Here's how the part is built. I have some questions about the finished solid (model axes, mm). A direction names the side the tool comes from. Round coordinates to 2 decimals unless told otherwise and drop trailing zeros. Write each loop counter-clockwise with the first axis right and the second up, starting at its lowest first coordinate (ties: lowest second). Pieces come first, ordered by that corner, then holes. Notation, with made-up numbers: (-26, -39.75) -> (26, -39.75) arc R34 cw to (26, -6.75) -> close; hole circle Ø9 at (11, 65). An arc over 180 degrees is marked (long way). Answer in a Markdown table with one row per item.
from build123d import *

# Parameters (mm, degrees)
F1_DEPTH = 7.5
F2_R     = 1.5
F3_DEPTH = 0.4910000058
F4_R     = 1.5
F5_DEPTH = 0.4910000058


with BuildPart() as f1:
    # F0 (on Right) → F1 (new body, symmetric)
    with BuildSketch(Plane.YZ):
        with BuildLine():
            Line((0, 0), (0, 30))
            ThreePointArc((0, 30), (-0.2450000029, 30.2450000029), (-0.4900000058, 30))
            Line((-0.4900000058, 30), (-0.4900000058, -0.4900000058))
            Line((-0.4900000058, -0.4900000058), (30, -0.4900000058))
            ThreePointArc((30, -0.4900000058), (30.2450000029, -0.2450000029), (30, 0))
            Line((30, 0), (0, 0))
        make_face()
    extrude(amount=F1_DEPTH, both=True)

    # F2 (on face) → F3 (cut, through all)
    with BuildSketch(Plane(origin=(0, 0, 0), x_dir=(-1, 0, 0), z_dir=(0, 1, 0))):
        with Locations((0, 20)):
            Circle(F2_R)
        with Locations((0, 10)):
            Circle(F2_R)
    extrude(amount=-F3_DEPTH, mode=Mode.SUBTRACT)

    # F4 (on face) → F5 (cut, through all)
    with BuildSketch(Plane.XY):
        with Locations((0, 20)):
            Circle(F4_R)
        with Locations((0, 10)):
            Circle(F4_R)
    extrude(amount=-F5_DEPTH, mode=Mode.SUBTRACT)


solid = f1.part
1) I want a section at D-D, the plane x = 3.25. List the corners of the cut face in (y, z) for me (3 decimals).
Response:
| item | result |
|---|---|
| outline | (-0.49, -0.49) -> (30, -0.49) arc R0.245 ccw to (30, 0) -> (0, 0) -> (0, 30) arc R0.245 ccw to (-0.49, 30) -> close |
2) I want a section at C-C, the plane x = 0. List the corners of the cut face in (y, z) for me (3 decimals), and give its area (3 significant figures).
Response:
| item | result |
|---|---|
| outline | (-0.49, -0.49) -> (8.5, -0.49) -> (8.5, 0) -> (0, 0) -> (0, 8.5) -> (-0.49, 8.5) -> close; (-0.49, 11.5) -> (0, 11.5) -> (0, 18.5) -> (-0.49, 18.5) -> close; (-0.49, 21.5) -> (0, 21.5) -> (0, 30) arc R0.245 ccw to (-0.49, 30) -> close; (11.5, -0.49) -> (18.5, -0.49) -> (18.5, 0) -> (11.5, 0) -> close; (21.5, -0.49) -> (30, -0.49) arc R0.245 ccw to (30, 0) -> (21.5, 0) -> close |
| area | 23.9 mm^2 |
3) We'd pull the mould along Y, two halves only. Please class faces 3 (the face through (-0.195, 21.487, -0.242)), 4 (the face through (0, -0.49, 15)), 5 (the face through (-0.325, 8.536, -0.242)), 6 (the face through (0, 15, -0.49)): +Y half, -Y half, draft (parallel to the pull), parting line (faces both ways), or undercut.
Response:
| item | result |
|---|---|
| face 3 | undercut |
| face 4 | -Y half |
| face 5 | undercut |
| face 6 | draft |
4) I want a section at A-A, the plane y = 20. List the corners of the cut face in (x, z) for me.
Response:
| item | result |
|---|---|
| outline | (-7.5, -0.49) -> (-1.5, -0.49) -> (-1.5, 0) -> (-7.5, 0) -> close; (1.5, -0.49) -> (7.5, -0.49) -> (7.5, 0) -> (1.5, 0) -> close |
5) I need wall thicknesses on line 1 (Y direction, x = 0, z = -0.25); line 2 (Z direction, x = 0.5, y = 27.5). Which ranges of each line are inside material? Lowest first, please. Write a range as [from, to].
Response:
| item | result |
|---|---|
| line 1 | y = [-0.49, 8.5], [11.5, 18.5], [21.5, 30.24] |
| line 2 | z = [-0.49, 0] |
6) Which directions (+Z, -Z, +X, -X, +Y, -Y) give clear straight access to the entire face, cutting with the end or side of a thin tool? Please do faces 1 (the face through (0, 15, 0)), 2 (the face through (0.195, -0.242, 21.487)).
Response:
| item | result |
|---|---|
| face 1 | +Z, +X, -X, +Y |
| face 2 | +Y, -Y |
7) For pin 1 (4 mm diameter, centred on x = 0, z = 20, fed in from +Y); pin 2 (1 mm diameter, centred on x = 5, y = 22.5, fed in from +Z); pin 3 (2.5 mm diameter, centred on x = 0, y = 20, fed in from +Z), each with a flat end and sliding along its axis, tell me the tip position at first contact or that it passes through.
Response:
| item | result |
|---|---|
| pin 1 | stops at y = 0 |
| pin 2 | stops at z = 0 |
| pin 3 | passes through |
